For this review, take the finished solid that the model builds, in its own axes (mm). A direction names the side the tool comes from. Give positions to 0.01 mm unless a question says otherwise; leave off trailing zeros. Order: outer loops, then holes, each group sorted by start corner. A loop starts at its lowest first (then second) coordinate and runs counter-clockwise, first axis right, second up. Notation, with made-up numbers: (63.25, 7) - (88.25, 7) arc R25 ccw to (88.25, 22) - close; hole circle Ø11 at (82, 26). An arc over 180 degrees is marked (long way). One line per item, written item: value.
```python
from build123d import *

# Parameters (mm, degrees)
BOX022_W               = 57.15
BOX022_H               = 19.05
BOX022_DEPTH           = 50.8
BOX023_W               = 60.325
BOX023_H               = 22.225
BOX023_DEPTH           = 52.3875
CUT025_PLACEMENT_ANGLE = 180


with BuildPart() as cube022:
    # Box022 → Box022 (new body)
    with BuildSketch(Plane(origin=(-28.575, -9.525, 0), x_dir=(1, 0, 0), z_dir=(0, 0, 1))):
        with Locations((28.575, 9.525)):
            Rectangle(BOX022_W, BOX022_H)
    extrude(amount=BOX022_DEPTH)


with BuildPart() as steel_cap001:
    # Box023 → Box023 (new body)
    with BuildSketch(Plane(origin=(-30.1625, -11.1125, -1.5875), x_dir=(1, 0, 0), z_dir=(0, 0, 1))):
        with Locations((30.1625, 11.1125)):
            Rectangle(BOX023_W, BOX023_H)
    extrude(amount=BOX023_DEPTH)

    # Cut025: cut Cube022
    add(cube022.part, mode=Mode.SUBTRACT)


with BuildPart() as steel_cap001_1:
    # Cut025 placement: moved
    add(steel_cap001.part.moved(Location((0, 0, 914.4))).rotate(Axis((0, 0, 914.4), (1, 0, 0)), CUT025_PLACEMENT_ANGLE))


solid = steel_cap001_1.part
```
(1) For P1, Ø5.5, axis at x = 11.5, y = 3, coming from the -Z side, flat-tipped, find the tip position at first contact; note if it passes through.
Answers below:
P1: stops at z = 914.4
(2) Take a section at A-A (y = 3). Write out the cut boundary in (x, z) (1 decimal), then the cut area to 3 significant figures.
Answers below:
outline: (-30.2, 863.6) - (-28.6, 863.6) - (-28.6, 914.4) - (28.6, 914.4) - (28.6, 863.6) - (30.2, 863.6) - (30.2, 916) - (-30.2, 916) - close
area: 257 mm^2
(3) Take a section at B-B (x = 9). Write out the cut boundary in (y, z) (1 decimal), then the cut area to 3 significant figures.
Answers below:
outline: (-11.1, 863.6) - (-9.5, 863.6) - (-9.5, 914.4) - (9.5, 914.4) - (9.5, 863.6) - (11.1, 863.6) - (11.1, 916) - (-11.1, 916) - close
area: 197 mm^2
(4) Take a section at C-C (z = 870). Write out the cut boundary in (x, y) (1 decimal).
Answers below:
outline: (-30.2, -11.1) - (30.2, -11.1) - (30.2, 11.1) - (-30.2, 11.1) - close; hole (-28.6, -9.5) - (28.6, -9.5) - (28.6, 9.5) - (-28.6, 9.5) - close
(5) Machinability: for faces 4 (the face through (0, 11.112, 890)), 5 (the face through (0, 0, 914.4)), which of the approach directions +Z, -Z, +X, -X, +Y, -Y give a long, thin tool a straight path to every point of the face, cutting with its end or side? Answer none if there is none.
Answers below:
face 4: +Z, -Z, +X, -X, +Y
face 5: -Z
(6) Wall thickness on line 1 (Y direction, x = 17, z = 901) (1 decimal); line 2 (X direction, y = 4.25, z = 890.5) (1 decimal); line 3 (Z direction, x = -13.5, y = -7.5): over which ranges is each line inside the solid? List them lowest first. Write a range as from..to.
Answers below:
line 1: y = -11.1..-9.5, 9.5..11.1
line 2: x = -30.2..-28.6, 28.6..30.2
line 3: z = 914.4..915.99
(7) Draft analysis for pull direction X (two halves, no side actions). For faces 1 (the face through (0, -11.113, 890)), 2 (the face through (-30.162, 0, 890)), 3 (the face through (0, -9.525, 889)), state which applies: pulls with the +X half, pulls with the -X half, needs draft (parallel to the pull), parting line crosses it, or undercut.
Answers below:
face 1: needs draft
face 2: pulls with the -X half
face 3: undercut
